from build123d import *

# Parameters (mm, degrees)
F0_W     = 141.246706
F0_H     = 98.03833
F0_W_2   = 126.943246
F0_H_2   = 86.714752
F1_DEPTH = 76.2
F2_R     = 12.513624
F3_DEPTH = 255.778
F4_W     = 67.345478
F4_H     = 38.1
F5_DEPTH = 172.466


with BuildPart() as f1:
    # F0 (on Top) → F1 (new body)
    with BuildSketch(Plane.XY):
        Rectangle(F0_W, F0_H)
        Rectangle(F0_W_2, F0_H_2, mode=Mode.SUBTRACT)
    extrude(amount=F1_DEPTH)

    # F2 (on face) → F3 (cut)
    with BuildSketch(Plane.YZ.offset(70.623353)):
        with Locations((0, 38.1)):
            Circle(F2_R)
    extrude(amount=-F3_DEPTH, mode=Mode.SUBTRACT)

    # F4 (on face) → F5 (cut)
    with BuildSketch(Plane.XZ.offset(49.019165)):
        with Locations((0, 57.15)):
            Rectangle(F4_W, F4_H)
    extrude(amount=-F5_DEPTH, mode=Mode.SUBTRACT)


solid = f1.part
Design review of the part built by this model. Coordinates are the model's own, in mm. A direction names the side the tool comes from. Coordinates: 2 decimals unless noted, no trailing zeros. Write each loop counter-clockwise with the first axis right and the second up, starting at its lowest first coordinate (ties: lowest second). Pieces come first, ordered by that corner, then holes. Notation, with made-up numbers: (36, 11.5) -> (58, 11.5) arc R25 ccw to (58, 38.5) -> close; hole circle Ø4 at (72, -17). An arc over 180 degrees is marked (long way). Write each question's results on one line, items separated by ' | '. Start each with the question number.
(1) Take a section at C-C on z = 7.5. Write out the cut boundary in (x, y), and give its area (3 significant figures).
(2) Take a section at B-B on x = 43.5. Write out the cut boundary in (y, z).
(3) For line 1 along X through (y, z) = (-24.5, 50); line 2 along Y through (x, z) = (50, 50); line 3 along Z through (x, y) = (67, 0), list the stretches that pass through material, from the lowest coordinate up. Write a range as from..to.
(4) Tool access review of faces 1 (the face through (-33.673, -46, 57)), 2 (the face through (-1, 49.019, 29)), 3 (the face through (-1, -43.357, 29)): name each direction out of +Z, -Z, +X, -X, +Y, -Y from which nothing blocks a thin tool from reaching the whole face with its end or side.
(5) Take a section at A-A on y = -35. Write out the cut boundary in (x, z), and give its area (3 significant figures).
(6) The part is to be moulded in two halves that separate along X. For faces 4 (the face through (-70.623, 10, 46)), 5 (the face through (-66.997, -1.629, 50.507)), 6 (the face through (-1, 43.357, 29)), say which applies: pulls with the +X half, pulls with the -X half, needs draft (parallel to the pull), parting line crosses it, or undercut.
(7) Take a section at D-D on y = 0. Write out the cut boundary in (x, z), and give its area (3 significant figures).
(8) Clearance check with flat-ended pins moving along their axes: P1, Ø5, axis at y = -5, z = 46.5, coming from the -X side; P2, Ø1.7, axis at x = -0.5, y = -45.5, coming from the +Z side. State where each tip first meets the part, or that it passes through.
Results found:
1) outline: (-70.62, -49.02) -> (70.62, -49.02) -> (70.62, 49.02) -> (-70.62, 49.02) -> close; hole (-63.47, -43.36) -> (63.47, -43.36) -> (63.47, 43.36) -> (-63.47, 43.36) -> close | area: 2,840 mm2
2) outline: (-49.02, 0) -> (-43.36, 0) -> (-43.36, 76.2) -> (-49.02, 76.2) -> close; (43.36, 0) -> (49.02, 0) -> (49.02, 76.2) -> (43.36, 76.2) -> close
3) line 1: x = -70.62..-63.47, 63.47..70.62 | line 2: y = -49.02..-43.36, 43.36..49.02 | line 3: z = 0..25.59, 50.61..76.2
4) face 1: +Z, +Y, -Y | face 2: +Z, -Z, +X, -X, +Y | face 3: +Z, -Z
5) outline: (-70.62, 0) -> (-63.47, 0) -> (-63.47, 76.2) -> (-70.62, 76.2) -> close; (63.47, 0) -> (70.62, 0) -> (70.62, 76.2) -> (63.47, 76.2) -> close | area: 1,090 mm2
6) face 4: pulls with the -X half | face 5: needs draft | face 6: undercut
7) outline: (-70.62, 0) -> (-63.47, 0) -> (-63.47, 25.59) -> (-70.62, 25.59) -> close; (-70.62, 50.61) -> (-63.47, 50.61) -> (-63.47, 76.2) -> (-70.62, 76.2) -> close; (63.47, 0) -> (70.62, 0) -> (70.62, 25.59) -> (63.47, 25.59) -> close; (63.47, 50.61) -> (70.62, 50.61) -> (70.62, 76.2) -> (63.47, 76.2) -> close | area: 732 mm2
8) P1: passes through | P2: stops at z = 38.1
